CAD build for the part. Positions are in the model's coordinates, mm. Give positions to 0.01 mm unless a question says otherwise; leave off trailing zeros. Loops run counter-clockwise (first coordinate to the right, second up) from the corner with the lowest first, then second, coordinate; pieces in that order, holes last. Notation, with made-up numbers: (75.5, 22) -> (118.5, 22) arc R31 ccw to (118.5, 47) -> close; hole circle Ø5 at (6.25, -30.5). An arc over 180 degrees is marked (long way). Use one line per item in the form item = value.
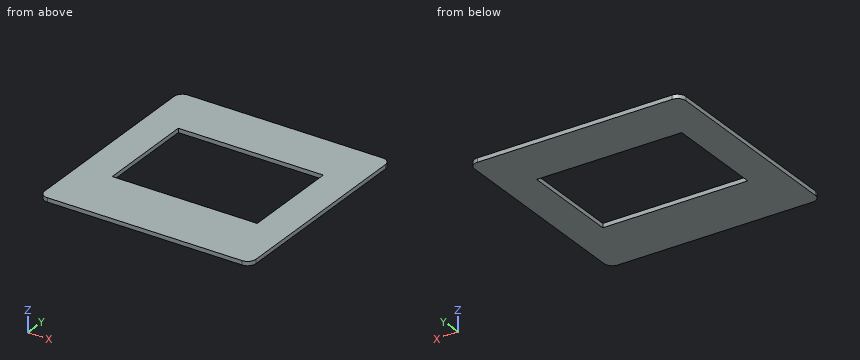
Autodesk Inventor part; units mm, degrees
ref_plane "YZ Plane" through (0, 0, 0) normal (1, 0, 0) x (0, 1, 0)
ref_plane "XZ Plane" through (0, 0, 0) normal (0, 1, 0) x (-1, 0, 0)
ref_plane "XY Plane" through (0, 0, 0) normal (0, 0, 1) x (1, 0, 0)
sketch "Skizze1" plane through (0, 0, 0) normal (0, 0, 1) x (1, 0, 0)
  line L0 (23.5, -25.5) -> (-23.5, -25.5)
  line L1 (-25.5, -23.5) -> (-25.5, 23.5)
  line L2 (-23.5, 25.5) -> (23.5, 25.5)
  line L3 (25.5, 23.5) -> (25.5, -23.5)
  line L4 (25.5, -25.5) -> (-25.5, 25.5) construction
  line L5 (-25.5, -25.5) -> (25.5, 25.5) construction
  line L6 (-17.5, 13) -> (17.5, 13)
  line L7 (17.5, 13) -> (17.5, -11)
  line L8 (17.5, -11) -> (-17.5, -11)
  line L9 (-17.5, -11) -> (-17.5, 13)
  line L10 (-17.5, 13) -> (17.5, -11) construction
  line L11 (17.5, 13) -> (-17.5, -11) construction
  arc A0 (-23.5, 25.5) -> (-25.5, 23.5) centre (-23.5, 23.5) ccw
  arc A1 (25.5, 23.5) -> (23.5, 25.5) centre (23.5, 23.5) ccw
  arc A2 (23.5, -25.5) -> (25.5, -23.5) centre (23.5, -23.5) ccw
  arc A3 (-25.5, -23.5) -> (-23.5, -25.5) centre (-23.5, -23.5) ccw
  point P0 (0, 0)
  point P1 (0, 1)
  dimension "d0" = 51
  dimension "d1" = 51
  dimension "d2" = 35
  dimension "d3" = 24
  dimension "d4" = 12.5
  dimension "d5" = 2
extrude "Extrusion1" add sketch "Skizze1" along normal blind 1
ref_plane "Arbeitsebene1" through (0, -23.5, 0) normal (1, 0, 0) x (0, 0, -1)
properties part number "00_Grating_1000linesPerMM"
1. Cut at B-B, the plane x = 13.5. Write the cut outline in (y, z).
Result sheet:
outline = (-25.5, 0) -> (-11, 0) -> (-11, 1) -> (-25.5, 1) -> close; (13, 0) -> (25.5, 0) -> (25.5, 1) -> (13, 1) -> close
2. Drill centre lines: line 1 (Y direction, x = 4.5, z = 0.5); line 2 (X direction, y = 11, z = 0.75). Where is each one in solid material? Low to high.
Result sheet:
line_1 = -25.5 to -11, 13 to 25.5
line_2 = -25.5 to -17.5, 17.5 to 25.5
3. Cut at A-A, the plane y = 3.5. Write the cut outline in (x, z).
Result sheet:
outline = (-25.5, 0) -> (-17.5, 0) -> (-17.5, 1) -> (-25.5, 1) -> close; (17.5, 0) -> (25.5, 0) -> (25.5, 1) -> (17.5, 1) -> close
4. Cut at C-C, the plane z = 0.55. Write the cut outline in (x, y).
Result sheet:
outline = (-25.5, -23.5) arc R2 ccw to (-23.5, -25.5) -> (23.5, -25.5) arc R2 ccw to (25.5, -23.5) -> (25.5, 23.5) arc R2 ccw to (23.5, 25.5) -> (-23.5, 25.5) arc R2 ccw to (-25.5, 23.5) -> close; hole (-17.5, -11) -> (17.5, -11) -> (17.5, 13) -> (-17.5, 13) -> close
